Verification items for the finished model (mm, model axes). Face numbers are marked on the shaded views. A direction names the side the tool comes from. Give positions to 0.01 mm unless a question says otherwise; leave off trailing zeros. Order: outer loops, then holes, each group sorted by start corner. A loop starts at its lowest first (then second) coordinate and runs counter-clockwise, first axis right, second up. Notation, with made-up numbers: (-17, 22) - (-10, 22) arc R22 cw to (-10, 51) - close; hole circle Ø5 at (-39, -20). An arc over 180 degrees is marked (long way). Answer as a JSON object with one key per item and string values.
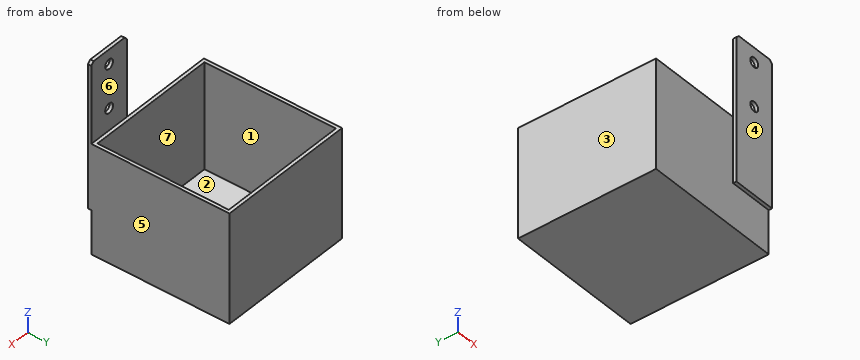
```python
from build123d import *

# Parameters (mm, degrees)
F0_W     = 27.7
F0_H     = 45
F0_W_2   = 2.3
F1_DEPTH = 2.3
F2_DEPTH = 95
F4_DEPTH = 72.7


with BuildPart() as f1:
    # F0 (on Front) → F1 (new body)
    with BuildSketch(Plane.XZ):
        with Locations((-90.369921, -12.07692)):
            Rectangle(F0_W, F0_H)
        Polygon((-76.519921, 10.42308), (-74.219921, 10.42308), (-74.219921, 63.42308), (-76.219921, 65.42308), (-102.219921, 65.42308), (-104.219921, 63.42308), (-104.219921, 10.42308), align=None)
        with BuildLine():
            ThreePointArc((-89.219921, 22.12308), (-91.553373, 23.089628), (-92.519921, 25.42308))
            ThreePointArc((-92.519921, 25.42308), (-91.553373, 27.756532), (-89.219921, 28.72308))
            ThreePointArc((-89.219921, 28.72308), (-86.886469, 27.756532), (-85.919921, 25.42308))
            ThreePointArc((-85.919921, 25.42308), (-86.886469, 23.089628), (-89.219921, 22.12308))
        make_face(mode=Mode.SUBTRACT)
        with BuildLine():
            ThreePointArc((-89.219921, 52.12308), (-91.553373, 53.089628), (-92.519921, 55.42308))
            ThreePointArc((-92.519921, 55.42308), (-91.553373, 57.756532), (-89.219921, 58.72308))
            ThreePointArc((-89.219921, 58.72308), (-86.886469, 57.756532), (-85.919921, 55.42308))
            ThreePointArc((-85.919921, 55.42308), (-86.886469, 53.089628), (-89.219921, 52.12308))
        make_face(mode=Mode.SUBTRACT)
        with Locations((-75.369921, -12.07692)):
            Rectangle(F0_W_2, F0_H)
    extrude(amount=F1_DEPTH)

    # F0 (on Front) → F2 (join)
    with BuildSketch(Plane.XZ):
        Polygon((-76.519921, -62.27692), (-76.519921, -34.57692), (-104.219921, -34.57692), (-104.219921, 10.42308), (-166.919921, 10.42308), (-166.919921, -62.27692), align=None)
        Polygon((-169.219921, -64.57692), (-74.219921, -64.57692), (-74.219921, -34.57692), (-76.519921, -34.57692), (-76.519921, -62.27692), (-166.919921, -62.27692), (-166.919921, 10.42308), (-169.219921, 10.42308), align=None)
        with Locations((-90.369921, -12.07692)):
            Rectangle(F0_W, F0_H)
        with Locations((-75.369921, -12.07692)):
            Rectangle(F0_W_2, F0_H)
    extrude(amount=-F2_DEPTH)

    # F3 (on face) → F4 (cut)
    with BuildSketch(Plane.XY.offset(10.42308)):
        Polygon((-104.219921, 2.3), (-76.519921, 2.3), (-76.519921, 92.7), (-166.919921, 92.7), (-166.919921, 2.3), align=None)
    extrude(amount=-F4_DEPTH, mode=Mode.SUBTRACT)


solid = f1.part
```
(1) Access from +Z, -Z, +X, -X, +Y, -Y to the whole of each face (thin tool, end or side, straight path). Record for the marked faces 5, 6 and 7.
Computed values:
{"face 5": "+Z, -Z, +X, +Y, -Y", "face 6": "+Z, +X, -X, +Y", "face 7": "+Z"}
(2) Section check B-B (y = 27). Record the cut outline in (x, z).
Computed values:
{"outline": "(-169.22, -64.58) - (-74.22, -64.58) - (-74.22, 10.42) - (-76.52, 10.42) - (-76.52, -62.28) - (-166.92, -62.28) - (-166.92, 10.42) - (-169.22, 10.42) - close"}
(3) Material ranges on line 1 along Y through (x, z) = (-153, 6.5); line 2 along X through (y, z) = (43.5, -21); line 3 along Z through (x, y) = (-135, 9.5), recorded low to high. Write a range as [from, to].
Computed values:
{"line 1": "y = [0, 2.3], [92.7, 95]", "line 2": "x = [-169.22, -166.92], [-76.52, -74.22]", "line 3": "z = [-64.58, -62.28]"}
(4) Gauge pin test, flat ends, axial feed: pin 1 Ø1.8 at (x, y) = (-92, -1) entering from -Z; pin 2 Ø22.5 at (x, z) = (-134.5, -20) entering from -Y; pin 3 Ø8 at (x, y) = (-136.5, 74) entering from +Z. Record the tip position at first contact, or that the pin passes through.
Computed values:
{"pin 1": "stops at z = -34.58", "pin 2": "stops at y = 0", "pin 3": "stops at z = -62.28"}
(5) Release check for a two-part mould opening along Y. For the marked faces 1, 2, 3 and 4 record: pulls with the +Y half, pulls with the -Y half, needs draft (parallel to the pull), parting line crosses it, or undercut.
Computed values:
{"face 1": "undercut", "face 2": "undercut", "face 3": "needs draft", "face 4": "pulls with the -Y half"}
(6) Section check D-D (z = 36). Record the cut outline in (x, y), then the cut area to 3 significant figures.
Computed values:
{"outline": "(-104.22, -2.3) - (-74.22, -2.3) - (-74.22, 0) - (-104.22, 0) - close", "area": "69.0 mm²"}
(7) Section check C-C (x = -130). Record the cut outline in (y, z).
Computed values:
{"outline": "(0, -64.58) - (95, -64.58) - (95, 10.42) - (92.7, 10.42) - (92.7, -62.28) - (2.3, -62.28) - (2.3, 10.42) - (0, 10.42) - close"}
(8) Section check A-A (z = -2.5). Record the cut outline in (x, y), then the cut area to 3 significant figures.
Computed values:
{"outline": "(-169.22, 0) - (-104.22, 0) - (-104.22, -2.3) - (-74.22, -2.3) - (-74.22, 95) - (-169.22, 95) - close; hole (-166.92, 2.3) - (-76.52, 2.3) - (-76.52, 92.7) - (-166.92, 92.7) - close", "area": "922 mm²"}
